Job drawing, mm, ordinate dimensions from the low corner. One solid piece. A direction names the side the tool comes from. Give positions to 0.01 mm unless a question says otherwise; leave off trailing zeros. Order: outer loops, then holes, each group sorted by start corner. A loop starts at its lowest first (then second) coordinate and runs counter-clockwise, first axis right, second up. Notation, with made-up numbers: (86, 33) - (105, 33) arc R19 ccw to (105, 42) - close; hole circle Ø9 at (59, 39.5). An arc over 180 degrees is marked (long way). Write each question's results on one line, items separated by ' | '. Start each with the question number.
1) Tool access for the marked faces 4 and 5: list every direction of +Z, -Z, +X, -X, +Y, -Y with a clear straight run to the whole face (end or side of a thin tool).
2) Two-plate mould, pull along Z, no slides. Class the marked faces 1, 2 and 3: +Z half, -Z half, draft (parallel to the pull), parting line (faces both ways), or undercut.
3) Cut at C-C on z = 9.25. List the corners of the cut face in (x, y), plus the area to 3 significant figures.
4) Drill centre lines: line 1 along Z through (x, y) = (14.75, 14.75); line 2 along Y through (x, z) = (10.6, 5.25); line 3 along Y through (x, z) = (10.6, 8.5). Where is each one in solid material? Low to high. Write a range as from..to.
5) Drop flat-ended pins along their axis: pin 1 Ø1 at (y, z) = (7.5, 4.5) entering from +X; pin 2 Ø8 at (x, y) = (10.6, 10.6) entering from -Z; pin 3 Ø6 at (y, z) = (16, 3) entering from +X; pin 4 Ø4 at (x, y) = (12, 7) entering from +Z. Give the stop position or say it passes through.
6) Cut at A-A on x = 10.6. List the corners of the cut face in (y, z).
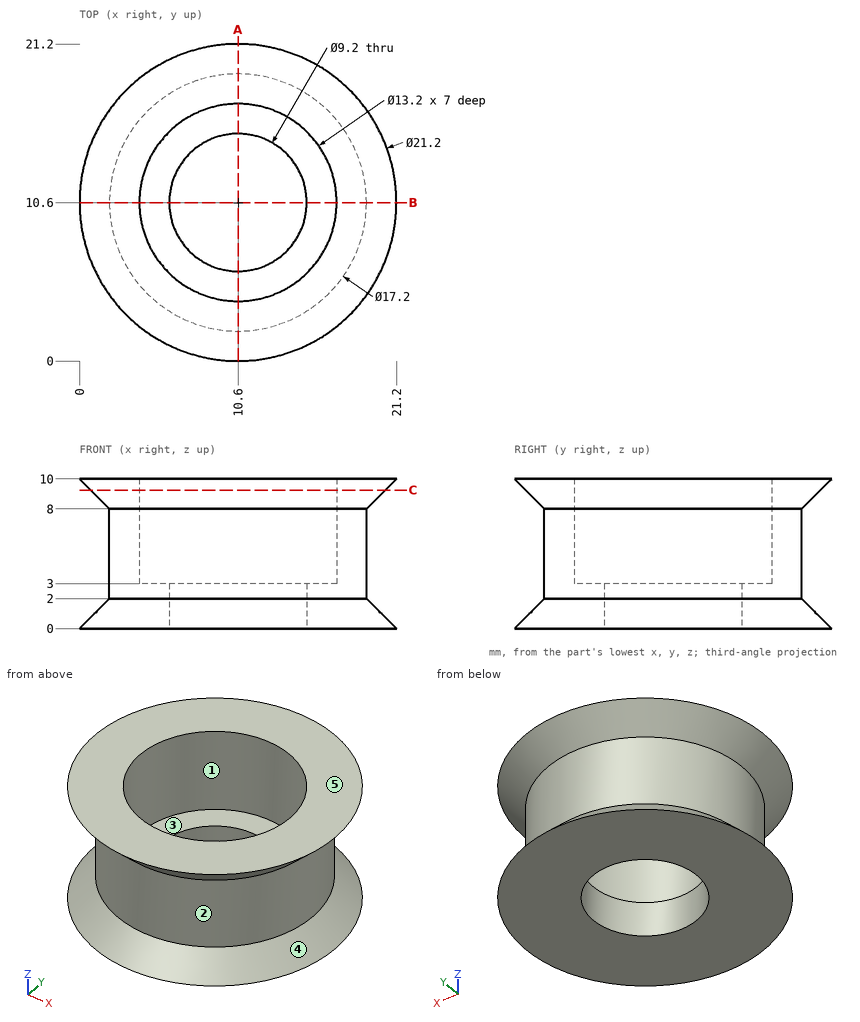
Results:
1) face 4: none | face 5: +Z, +X, -X, +Y, -Y
2) face 1: draft | face 2: undercut | face 3: +Z half
3) outline: circle Ø19.7 at (10.6, 10.6); hole circle Ø13.2 at (10.6, 10.6) | area: 168 mm^2
4) line 1: 0..3 | line 2: 2..4, 17.2..19.2 | line 3: 1.5..4, 17.2..19.7
5) pin 1: x = 18.8 | pin 2: through | pin 3: x = 20.06 | pin 4: z = 3
6) outline: (0, 0) - (6, 0) - (6, 3) - (4, 3) - (4, 10) - (0, 10) - (2, 8) - (2, 2) - close; (15.2, 0) - (21.2, 0) - (19.2, 2) - (19.2, 8) - (21.2, 10) - (17.2, 10) - (17.2, 3) - (15.2, 3) - close
